The listing builds one solid part. Answer for the finished solid, in the listing's coordinates (mm). A direction names the side the tool comes from. Round coordinates to 2 decimals unless told otherwise and drop trailing zeros. Loops run counter-clockwise (first coordinate to the right, second up) from the corner with the lowest first, then second, coordinate; pieces in that order, holes last. Notation, with made-up numbers: (63, 50.5) - (73, 50.5) arc R5 cw to (73, 55.5) - close; hole circle Ø7 at (13, -4). An arc over 180 degrees is marked (long way). One line per item, written item: value.
```python
from build123d import *

# Parameters (mm, degrees)
SKETCH_1_W          = 45
SKETCH_1_H          = 61
SKETCH_1_W_2        = 42
SKETCH_1_H_2        = 58
SKETCH_1_R          = 1.55
EXTRUDE_1_DEPTH     = 13
EXTRUDE_2_DEPTH     = 1
SKETCH_1_4_W        = 11
SKETCH_1_4_H        = 33
EXTRUDE_3_DEPTH     = 4.5
SKETCH_1_5_W        = 14.30710185
SKETCH_1_5_H        = 23
EXTRUDE_4_DEPTH     = 6.5
SKETCH_1_6_W        = 2
SKETCH_1_6_H        = 15
EXTRUDE_5_DEPTH     = 10
SKETCH_1_8_W        = 1.5
SKETCH_1_8_H        = 33
EXTRUDE_6_DEPTH     = 8
SKETCH_2_W          = 10.357609848
SKETCH_2_H          = 23.284426604
CUT_EXTRUDE_1_DEPTH = 2.5


with BuildPart() as part:
    # Sketch 1 → Extrude 1 (new body)
    # profile 1 of 2: a face of its own
    with BuildSketch(Plane.XY):
        Rectangle(SKETCH_1_W, SKETCH_1_H)
        Rectangle(SKETCH_1_W_2, SKETCH_1_H_2, mode=Mode.SUBTRACT)
    # profile 2 of 2: a face of its own
    with BuildSketch(Plane.XY):
        Polygon((27.5, -24.5), (22.5, -19.601020514), (22.5, -30.5), (27.5, -30.5), align=None)
        with Locations((25, -27.5)):
            Circle(SKETCH_1_R, mode=Mode.SUBTRACT)
    extrude(amount=-EXTRUDE_1_DEPTH)

    # Sketch 1_3 → Extrude 2 (add)
    with BuildSketch(Plane.XY):
        Polygon((-21, -29), (4.230409418, -29), (4.230409418, 4), (4.230409418, 29), (-21, 29), align=None)
    extrude(amount=-EXTRUDE_2_DEPTH)

    # Sketch 1_4 → Extrude 3 (add)
    with BuildSketch(Plane.XY):
        with Locations((9.730409418, -12.5)):
            Rectangle(SKETCH_1_4_W, SKETCH_1_4_H)
    extrude(amount=-EXTRUDE_3_DEPTH)

    # Sketch 1_5 → Extrude 4 (add)
    with BuildSketch(Plane.XY):
        with Locations((13.846449075, 17.5)):
            Rectangle(SKETCH_1_5_W, SKETCH_1_5_H)
    extrude(amount=-EXTRUDE_4_DEPTH)

    # Sketch 1_6 → Extrude 5 (add)
    with BuildSketch(Plane.XY):
        Polygon((16.730409418, 5), (21, 5), (21, 6), (6.69289815, 6), (6.69289815, 29), (4.230409418, 29), (4.230409418, 4), (15.230409418, 4), (16.730409418, 4), align=None)
        with Locations((20, -21.5)):
            Rectangle(SKETCH_1_6_W, SKETCH_1_6_H)
    extrude(amount=-EXTRUDE_5_DEPTH)

    # Sketch 1_8 → Extrude 6 (add)
    with BuildSketch(Plane.XY):
        with Locations((15.980409418, -12.5)):
            Rectangle(SKETCH_1_8_W, SKETCH_1_8_H)
    extrude(amount=-EXTRUDE_6_DEPTH)

    # Sketch 2 → Cut-Extrude 1 (cut, symmetric)
    with BuildSketch(Plane.ZY.offset(-21)):
        with Locations((-7.821195076, -6.642213302)):
            Rectangle(SKETCH_2_W, SKETCH_2_H)
    extrude(amount=CUT_EXTRUDE_1_DEPTH, both=True, mode=Mode.SUBTRACT)


solid = part.part
```
1) For faces 4 (the flat face through (19, -23, -5)), 5 (the flat face through (22.5, 11, -5)), 6 (the flat face through (10, -12, -4.5)), 7 (the flat face through (21, -18.284, -7)), determine the directions among +Z, -Z, +X, -X, +Y, -Y from which every point of the face is accessible in a straight line to the end or side of a thin tool.
Final values:
face 4: +Z, -Z
face 5: +Z, -Z, +X, +Y
face 6: -Z
face 7: -Z, +X
2) A cutting plane is placed at D-D on z = -3.5. Give the vertices of the cut face in (x, y).
Final values:
outline: (-22.5, -30.5) - (27.5, -30.5) - (27.5, -24.5) - (22.5, -19.6) - (22.5, -18.28) - (19, -18.28) - (19, -29) - (16.73, -29) - (16.73, 5) - (22.5, 5) - (22.5, 30.5) - (-22.5, 30.5) - close; hole (-21, -29) - (4.23, -29) - (4.23, 29) - (-21, 29) - close; hole circle Ø3.1 at (25, -27.5)
3) For a pull along X with two mould halves and no side action, classify faces 1 (the flat face through (27.5, -28, -6)), 2 (the flat face through (-3, 0, 0)), 3 (the flat face through (-9, 0, -1)) as released by +X, released by -X, zero draft, split by the parting line, or undercut.
Final values:
face 1: released by +X
face 2: zero draft
face 3: undercut
4) Consider L1, parallel to X at y = 24, z = -9.25; L2, parallel to Y at x = 1.5, z = -2; L3, parallel to X at y = 23, z = -6.25. Determine where each line is inside the solid, lowest interval first.
Final values:
L1: -22.5 to -21, 4.23 to 6.69, 21 to 22.5
L2: -30.5 to -29, 29 to 30.5
L3: -22.5 to -21, 4.23 to 22.5
5) A cutting plane is placed at A-A on y = -27.5. Give the vertices of the cut face in (x, z).
Final values:
outline: (-22.5, -13) - (-21, -13) - (-21, -1) - (4.23, -1) - (4.23, -4.5) - (15.23, -4.5) - (15.23, -8) - (16.73, -8) - (16.73, 0) - (-22.5, 0) - close; (19, -10) - (21, -10) - (21, -13) - (23.45, -13) - (23.45, 0) - (19, 0) - close; (26.55, -13) - (27.5, -13) - (27.5, 0) - (26.55, 0) - close
6) A cutting plane is placed at B-B on y = 2. Give the vertices of the cut face in (x, z), and give its area (3 significant figures).
Final values:
outline: (-22.5, -13) - (-21, -13) - (-21, -1) - (4.23, -1) - (4.23, -4.5) - (15.23, -4.5) - (15.23, -8) - (16.73, -8) - (16.73, 0) - (-22.5, 0) - close; (21, -2.64) - (22.5, -2.64) - (22.5, 0) - (21, 0) - close
area: 110 mm2
7) A cutting plane is placed at C-C on x = 17.5. Give the vertices of the cut face in (y, z), and give its area (4 significant figures).
Final values:
outline: (-30.5, -13) - (-29, -13) - (-29, 0) - (-30.5, 0) - close; (5, -10) - (6, -10) - (6, -6.5) - (29, -6.5) - (29, -13) - (30.5, -13) - (30.5, 0) - (5, 0) - close
area: 198.5 mm2
8) Each of these flat-tipped pins is pushed along its axis until it touches: pin 1 Ø5 at (x, y) = (13.5, 22) entering from -Z; pin 2 Ø3 at (y, z) = (-8.5, -4) entering from +X; pin 3 Ø2 at (y, z) = (-13.5, -8.5) entering from +X. Where does it stop, or does it pass through?
Final values:
pin 1: z = -6.5
pin 2: x = 22.5
pin 3: x = 16.73
